```python
from build123d import *

# Parameters (mm, degrees)
CROQUIS1_R                   = 5.8
SALIENTE_EXTRUIR1_DEPTH      = 32.5
CORTAR_EXTRUIR1_DEPTH        = 24
CORTAR_EXTRUIR_L_MINA1_START = -6.5
CROQUIS3_R                   = 5.8
CROQUIS3_R_2                 = 5
CORTAR_EXTRUIR_L_MINA1_DEPTH = 3
CROQUIS4_W                   = 7
CROQUIS4_H                   = 7
SALIENTE_EXTRUIR2_DEPTH      = 7
CROQUIS6_R                   = 1.75
CORTAR_EXTRUIR3_DEPTH        = 10.3
CORTAR_EXTRUIR4_DEPTH        = 18


with BuildPart() as part:
    # Croquis1 → Saliente-Extruir1 (new body, symmetric)
    with BuildSketch(Plane.XY):
        Circle(CROQUIS1_R)
    extrude(amount=SALIENTE_EXTRUIR1_DEPTH, both=True)

    # Croquis2 → Cortar-Extruir1 (cut)
    with BuildSketch(Plane.XY):
        with BuildLine():
            Line((-5.8, 0), (5.8, 0))
            ThreePointArc((5.8, 0), (0, 5.8), (-5.8, 0))
        make_face()
    extrude(amount=-CORTAR_EXTRUIR1_DEPTH, mode=Mode.SUBTRACT)

    # Croquis3 → Cortar-Extruir-L_mina1 (cut)
    with BuildSketch(Plane.XY.offset(32.5).offset(CORTAR_EXTRUIR_L_MINA1_START)):
        Circle(CROQUIS3_R)
        Circle(CROQUIS3_R_2, mode=Mode.SUBTRACT)
    extrude(amount=-CORTAR_EXTRUIR_L_MINA1_DEPTH, mode=Mode.SUBTRACT)

    # Croquis4 → Saliente-Extruir2 (add)
    with BuildSketch(Plane.XY.offset(32.5)):
        Rectangle(CROQUIS4_W, CROQUIS4_H)
    extrude(amount=SALIENTE_EXTRUIR2_DEPTH)

    # Croquis6 → Cortar-Extruir3 (cut, through all)
    with BuildSketch(Plane.ZY.offset(3.5)):
        with Locations((36.5, 0)):
            Circle(CROQUIS6_R)
    extrude(amount=-CORTAR_EXTRUIR3_DEPTH, mode=Mode.SUBTRACT)

    # Croquis2_2 → Cortar-Extruir4 (cut)
    with BuildSketch(Plane.XY):
        with BuildLine():
            Line((-5.8, 0), (5.8, 0))
            ThreePointArc((5.8, 0), (0, 5.8), (-5.8, 0))
        make_face()
    extrude(amount=CORTAR_EXTRUIR4_DEPTH, mode=Mode.SUBTRACT)


solid = part.part
```
Design review of the part built by this model. Coordinates are the model's own, in mm. A direction names the side the tool comes from. Give positions to 0.01 mm unless a question says otherwise; leave off trailing zeros. Write each loop counter-clockwise with the first axis right and the second up, starting at its lowest first coordinate (ties: lowest second). Pieces come first, ordered by that corner, then holes. Notation, with made-up numbers: (38.25, 27.25) - (87.25, 27.25) arc R21 cw to (87.25, 63.25) - close; hole circle Ø5 at (23, -1.5). An arc over 180 degrees is marked (long way). Return JSON: item names as keys, results as strings. Group by question number.
(1) Mouldability with a two-part tool opening along Y and no side actions: class faces 1 (the flat face through (2, 5, 23)), 2 (the cylindrical face through (-0.049, -0.67, 38.117)), 3 (the flat face through (0, 3.5, 36)), 4 (the cylindrical face through (-5.794, 0.255, 29.296)) as +Y half, -Y half, draft (parallel to the pull), parting line (faces both ways), or undercut.
(2) Machinability: for faces 5 (the flat face through (0, 2, 18)), 6 (the cylindrical face through (-1.08, -4.88, 24.52)), 7 (the flat face through (0, -3.5, 36)), 8 (the flat face through (3.5, 0, 34)), which of the approach directions +Z, -Z, +X, -X, +Y, -Y give a long, thin tool a straight path to every point of the face, cutting with its end or side? Answer none if there is none.
(3) We need section D-D, the plane z = 24.5. Give the boundary of the cut face in (x, y), then the cut area to 3 significant figures.
(4) We need section B-B, the plane x = 0. Give the boundary of the cut face in (y, z).
(5) To check wall thickness, follow probe 1 along Z at (x, y) = (-5, 2); probe 2 along Y at (x, z) = (-1.5, 36.5); probe 3 along Z at (x, y) = (2, 2). State the ranges of each line that lie inside material, in increasing order.
(6) We need section A-A, the plane z = 36.5. Give the boundary of the cut face in (x, y).
(7) We need section C-C, the plane x = -4.25. Give the boundary of the cut face in (y, z).
(8) Insertion check: pin 1 (3.5 mm diameter, centred on x = -0.5, z = 34.5, fed in from -Y); pin 2 (1 mm diameter, centred on y = 2.5, z = 29, fed in from +X); pin 3 (2 mm diameter, centred on y = -1, z = 35, fed in from -X). Each pin has a flat end and moves straight along its axis. Give the tip position at first contact, or say it passes through.
Reported:
{
 "1": {"face 1": "draft", "face 2": "undercut", "face 3": "+Y half", "face 4": "parting line"},
 "2": {"face 5": "+X, -X, +Y", "face 6": "none", "face 7": "+Z, +X, -X, -Y", "face 8": "+Z, +X, +Y, -Y"},
 "3": {"outline": "circle Ø10 at (0, 0)", "area": "78.5 mm2"},
 "4": {"outline": "(-5.8, -32.5) - (5.8, -32.5) - (5.8, -24) - (0, -24) - (0, 18) - (5.8, 18) - (5.8, 23) - (5, 23) - (5, 26) - (5.8, 26) - (5.8, 32.5) - (3.5, 32.5) - (3.5, 39.5) - (-3.5, 39.5) - (-3.5, 32.5) - (-5.8, 32.5) - (-5.8, 26) - (-5, 26) - (-5, 23) - (-5.8, 23) - close; hole circle Ø3.5 at (0, 36.5)"},
 "5": {"probe 1": "z = -32.5 to -24, 18 to 23, 26 to 32.5", "probe 2": "y = -3.5 to -1.75, 1.75 to 3.5", "probe 3": "z = -32.5 to -24, 18 to 39.5"},
 "6": {"outline": "(-3.5, -3.5) - (3.5, -3.5) - (3.5, -1.75) - (-3.5, -1.75) - close; (-3.5, 1.75) - (3.5, 1.75) - (3.5, 3.5) - (-3.5, 3.5) - close"},
 "7": {"outline": "(-3.95, -32.5) - (3.95, -32.5) - (3.95, -24) - (0, -24) - (0, 18) - (3.95, 18) - (3.95, 23) - (2.63, 23) - (2.63, 26) - (3.95, 26) - (3.95, 32.5) - (-3.95, 32.5) - (-3.95, 26) - (-2.63, 26) - (-2.63, 23) - (-3.95, 23) - close"},
 "8": {"pin 1": "stops at y = -3.5", "pin 2": "stops at x = 5.44", "pin 3": "stops at x = -3.5"}
}
